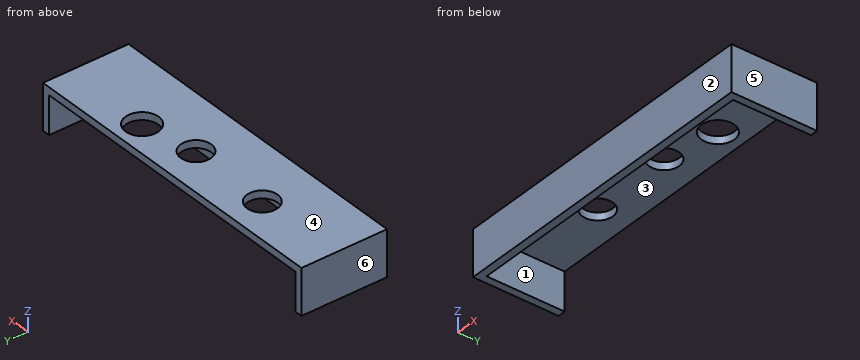
```python
from build123d import *

# Parameters (mm, degrees)
SKETCH_1_W      = 128
SKETCH_1_H      = 33.7
SKETCH_1_R      = 6.5
SKETCH_1_R_2    = 6
EXTRUDE_1_DEPTH = 3
EXTRUDE_2_DEPTH = 15


with BuildPart() as part:
    # 草圖1 → 填料-伸長1 (new body)
    with BuildSketch(Plane.XY):
        with Locations((-30.980810071, -55.280072207)):
            Rectangle(SKETCH_1_W, SKETCH_1_H)
        with Locations((-3.480809972, -48.430072207)):
            Circle(SKETCH_1_R, mode=Mode.SUBTRACT)
        with Locations((-25.269668394, -52.330072207)):
            Circle(SKETCH_1_R_2, mode=Mode.SUBTRACT)
        with Locations((-59.319668394, -51.380072207)):
            Circle(SKETCH_1_R_2, mode=Mode.SUBTRACT)
    extrude(amount=EXTRUDE_1_DEPTH)

    # 草圖2 → 填料-伸長2 (add)
    with BuildSketch(Plane(origin=(0, 0, 0), x_dir=(-1, 0, 0), z_dir=(0, 0, -1))):
        Polygon((91.980810071, -38.430072207), (91.980810071, -69.130072207), (-30.019189929, -69.130072207), (-30.019189929, -38.430072207), (-33.019189929, -38.430072207), (-33.019189929, -72.130072207), (94.980810071, -72.130072207), (94.980810071, -38.430072207), align=None)
    extrude(amount=EXTRUDE_2_DEPTH)


solid = part.part
```
Could you check a few things on this model? Use its own coordinates, in mm. Face numbers are marked on the shaded views. A direction names the side the tool comes from. Round coordinates to 2 decimals unless told otherwise and drop trailing zeros. Loops run counter-clockwise (first coordinate to the right, second up) from the corner with the lowest first, then second, coordinate; pieces in that order, holes last. Notation, with made-up numbers: (-23, 9.25) - (19, 9.25) arc R21 cw to (19, 27.25) - close; hole circle Ø10 at (4, -15). An arc over 180 degrees is marked (long way). Answer in a Markdown table with one row per item. Add a question column.
(1) I need wall thicknesses on line 1 along X through (y, z) = (-65, -11.75); line 2 along X through (y, z) = (-46, 0.5); line 3 along Y through (x, z) = (-62.5, -13.5). Which ranges of each line are inside material? Lowest first, please.
(2) I'm going to push flat-ended pins straight in: pin 1 (9 mm diameter, centred on x = -53.5, y = -47.5, fed in from -Z); pin 2 (7.5 mm diameter, centred on x = -4, z = -9, fed in from +Y); pin 3 (10.5 mm diameter, centred on x = -3.48, y = -48.43, fed in from +Z). Where does each tip first touch, or does it pass through?
(3) If we mould it in two halves opening along X, with no side actions, what happens to the marked faces 3, 4, 5 and 6? For each: pulls with the +X half, pulls with the -X half, needs draft (parallel to the pull), parting line crosses it, or undercut.
(4) If we section it at C-C (z = -4.75): Please give me the cut outline in (x, y), plus the area to 3 significant figures.
(5) For the marked faces 1 and 2, which set-ups out of +Z, -Z, +X, -X, +Y, -Y let a thin tool reach every point of the face, with its end or its side?
(6) If we section it at D-D (z = 1.5): Please give me the cut outline in (x, y).
(7) If we section it at B-B (x = -26): Please give me the cut outline in (y, z), plus the area to 3 significant figures.
(8) If we section it at A-A (y = -66): Please give me the cut outline in (x, z).
Model answer:
| question | item | result |
|---|---|---|
| 1 | line 1 | x = -94.98 to -91.98, 30.02 to 33.02 |
| 1 | line 2 | x = -94.98 to -61.98, -56.66 to -9.51, 2.55 to 33.02 |
| 1 | line 3 | y = -72.13 to -69.13 |
| 2 | pin 1 | stops at z = 0 |
| 2 | pin 2 | stops at y = -69.13 |
| 2 | pin 3 | passes through |
| 3 | face 3 | undercut |
| 3 | face 4 | needs draft |
| 3 | face 5 | pulls with the +X half |
| 3 | face 6 | pulls with the -X half |
| 4 | outline | (-94.98, -72.13) - (33.02, -72.13) - (33.02, -38.43) - (30.02, -38.43) - (30.02, -69.13) - (-91.98, -69.13) - (-91.98, -38.43) - (-94.98, -38.43) - close |
| 4 | area | 568 mm² |
| 5 | face 1 | -Z, +Y |
| 5 | face 2 | +Z, -Z, +X, -X, -Y |
| 6 | outline | (-94.98, -72.13) - (33.02, -72.13) - (33.02, -38.43) - (-94.98, -38.43) - close; hole circle Ø12 at (-59.32, -51.38); hole circle Ø12 at (-25.27, -52.33); hole circle Ø13 at (-3.48, -48.43) |
| 7 | outline | (-72.13, -15) - (-69.13, -15) - (-69.13, 0) - (-58.29, 0) - (-58.29, 3) - (-72.13, 3) - close; (-46.37, 0) - (-38.43, 0) - (-38.43, 3) - (-46.37, 3) - close |
| 7 | area | 110 mm² |
| 8 | outline | (-94.98, -15) - (-91.98, -15) - (-91.98, 0) - (30.02, 0) - (30.02, -15) - (33.02, -15) - (33.02, 3) - (-94.98, 3) - close |
